Geometry: final body of the model. Coordinates: model frame, mm. A direction names the side the tool comes from. Give positions to 0.01 mm unless a question says otherwise; leave off trailing zeros. Loops run counter-clockwise (first coordinate to the right, second up) from the corner with the lowest first, then second, coordinate; pieces in that order, holes last.
Autodesk Inventor part; units mm, degrees
ref_plane "YZ Plane" through (0, 0, 0) normal (1, 0, 0) x (0, 1, 0)
ref_plane "XZ Plane" through (0, 0, 0) normal (0, 1, 0) x (-1, 0, 0)
ref_plane "XY Plane" through (0, 0, 0) normal (0, 0, 1) x (1, 0, 0)
sketch "スケッチ1" plane through (0, 0, 0) normal (0, 0, 1) x (1, 0, 0)
  line L0 (7.25, -16) -> (-7.25, -16)
  line L1 (-16.25, -16) -> (-16.25, 16)
  line L2 (-7.25, 16) -> (7.25, 16)
  line L3 (16.25, -16) -> (-16.25, 16) construction
  line L4 (-16.25, -16) -> (16.25, 16) construction
  line L5 (16.25, 0) -> (46.25, 0) construction
  line L6 (46.25, -10.5) -> (16.25, -10.5) construction
  line L7 (16.25, 10.5) -> (46.25, 10.5) construction
  line L8 (46.25, 10.5) -> (46.25, -10.5) construction
  line L9 (46.25, -10.5) -> (16.25, 10.5) construction
  line L10 (16.25, -10.5) -> (46.25, 10.5) construction
  line L11 (46.25, 11.5) -> (15.25, 11.5)
  line L12 (15.25, 11.5) -> (15.25, -11.5)
  line L13 (15.25, -11.5) -> (46.25, -11.5)
  line L14 (46.25, 19.5) -> (7.25, 19.5)
  line L15 (7.25, -19.5) -> (46.25, -19.5)
  line L16 (46.25, 11.5) -> (46.25, 19.5)
  line L17 (46.25, -11.5) -> (46.25, -19.5)
  line L18 (16.25, 10.5) -> (16.25, -10.5) construction
  line L19 (7.25, 19.5) -> (7.25, 16)
  line L20 (7.25, -16) -> (7.25, -19.5)
  line L21 (-16.25, -16) -> (-16.25, -26)
  line L22 (-16.25, -26) -> (-7.25, -26)
  line L23 (-7.25, 26) -> (-16.25, 26)
  line L24 (-16.25, 26) -> (-16.25, 16)
  line L25 (-11.75, 26) -> (-11.75, -26) construction
  line L26 (-11.75, 0) -> (-16.25, 0) construction
  circle A0 centre (-11.75, -21) radius 1.6
  line L27 (-7.25, -26) -> (-7.25, -16)
  line L28 (-7.25, 16) -> (-7.25, 26)
  circle A1 centre (-11.75, 21) radius 1.6
  line L29 (46.25, 10.5) -> (16.25, 10.5) construction
  line L30 (31.25, 10.5) -> (31.25, 19.5) construction
  line L31 (31.25, 15) -> (46.25, 15) construction
  circle A2 centre (37.05, 15) radius 1.6 construction
  circle A3 centre (42.25, 15) radius 1.6
  circle A4 centre (25.45, 15) radius 1.6 construction
  circle A5 centre (20.25, 15) radius 1.6
  circle A6 centre (37.05, -15) radius 1.6 construction
  circle A7 centre (42.25, -15) radius 1.6
  circle A8 centre (25.45, -15) radius 1.6 construction
  circle A9 centre (20.25, -15) radius 1.6
  point P0 (0, 0)
  point P1 (31.25, 0)
  dimension "d21" = 32.5
  dimension "d22" = 32
  dimension "d24" = 30
  dimension "d25" = 21
  dimension "d26" = 1
  dimension "d28" = 30
  dimension "d30" = 9
  dimension "d32" = 9
  dimension "d33" = 3.2
  dimension "d34" = 5
  dimension "d35" = 10
  dimension "d36" = 8
  dimension "d37" = 31
  dimension "d38" = 3.5
  dimension "d39" = 35.5
  dimension "d40" = 9
  dimension "d41" = 3.2
  dimension "d42" = 3.2
  dimension "d43" = 4
  dimension "d44" = 31
  dimension "d46" = 2
extrude "押し出し1" add sketch "スケッチ1" along normal blind 3
fillet "フィレット1" radius 2 10 edges at (7.25, 19.5, 1.5) (-7.25, 26, 1.5) (-16.25, 26, 1.5) (46.25, 19.5, 1.5) (46.25, 11.5, 1.5) (46.25, -11.5, 1.5) (46.25, -19.5, 1.5) (7.25, -19.5, 1.5) (-7.25, -26, 1.5) (-16.25, -26, 1.5)
fillet "フィレット2" radius 3 6 edges at (15.25, -11.5, 1.5) (15.25, 11.5, 1.5) (7.25, 16, 1.5) (7.25, -16, 1.5) (-7.25, -16, 1.5) (-7.25, 16, 1.5)
sketch "スケッチ2" plane through (0, 0, 3) normal (0, 0, 1) x (1, 0, 0)
  arc A0 (-16.25, -24) -> (-14.25, -26) centre (-14.25, -24) ccw
  line L0 (-14.25, -26) -> (-9.25, -26)
  arc A1 (-9.25, -26) -> (-7.25, -24) centre (-9.25, -24) ccw
  line L1 (-7.25, -24) -> (-7.25, -19)
  arc A2 (-4.25, -16) -> (-7.25, -19) centre (-4.25, -19) ccw
  line L2 (-4.25, -16) -> (4.4803, -16)
  arc A3 (7.3421, -18.1) -> (4.4803, -16) centre (4.4803, -19) ccw
  arc A4 (7.3421, -18.1) -> (9.25, -19.5) centre (9.25, -17.5) ccw
  line L3 (9.25, -19.5) -> (44.25, -19.5)
  arc A5 (44.25, -19.5) -> (46.25, -17.5) centre (44.25, -17.5) ccw
  line L4 (46.25, -17.5) -> (46.25, -13.5)
  arc A6 (46.25, -13.5) -> (44.25, -11.5) centre (44.25, -13.5) ccw
  line L5 (44.25, -11.5) -> (18.25, -11.5)
  arc A7 (15.25, -8.5) -> (18.25, -11.5) centre (18.25, -8.5) ccw
  line L6 (15.25, -8.5) -> (15.25, 8.5)
  arc A8 (18.25, 11.5) -> (15.25, 8.5) centre (18.25, 8.5) ccw
  line L7 (18.25, 11.5) -> (44.25, 11.5)
  arc A9 (44.25, 11.5) -> (46.25, 13.5) centre (44.25, 13.5) ccw
  line L8 (46.25, 13.5) -> (46.25, 17.5)
  arc A10 (46.25, 17.5) -> (44.25, 19.5) centre (44.25, 17.5) ccw
  line L9 (44.25, 19.5) -> (9.25, 19.5)
  arc A11 (9.25, 19.5) -> (7.3421, 18.1) centre (9.25, 17.5) ccw
  arc A12 (4.4803, 16) -> (7.3421, 18.1) centre (4.4803, 19) ccw
  line L10 (4.4803, 16) -> (-4.25, 16)
  arc A13 (-7.25, 19) -> (-4.25, 16) centre (-4.25, 19) ccw
  line L11 (-7.25, 19) -> (-7.25, 24)
  arc A14 (-7.25, 24) -> (-9.25, 26) centre (-9.25, 24) ccw
  line L12 (-9.25, 26) -> (-14.25, 26)
  arc A15 (-14.25, 26) -> (-16.25, 24) centre (-14.25, 24) ccw
  line L13 (-16.25, 24) -> (-16.25, -24)
  circle A16 centre (42.25, -15) radius 1.6
  circle A17 centre (20.25, -15) radius 1.6
  circle A18 centre (20.25, 15) radius 1.6
  circle A19 centre (42.25, 15) radius 1.6
  circle A20 centre (-11.75, 21) radius 1.6
  circle A21 centre (-11.75, -21) radius 1.6
  circle A22 centre (-11.75, 21) radius 4.6
  circle A23 centre (-11.75, -21) radius 4.6
  line L14 (4.4803, -13) -> (-4.25, -13)
  arc A24 (-9.8384, -16.816) -> (-10.25, -19) centre (-4.25, -19) ccw
  line L15 (-10.25, -19) -> (-10.25, -23)
  line L16 (-10.25, -23) -> (-13.25, -23)
  line L17 (-13.25, 23) -> (-10.25, 23)
  line L18 (-10.25, 23) -> (-10.25, 19)
  arc A25 (-10.25, 19) -> (-9.8384, 16.816) centre (-4.25, 19) ccw
  line L19 (-4.25, 13) -> (4.4803, 13)
  line L20 (9.9347, 16.5) -> (43.25, 16.5)
  line L21 (43.25, 16.5) -> (43.25, 14.5)
  line L22 (43.25, 14.5) -> (18.25, 14.5)
  line L23 (12.25, 8.5) -> (12.25, -8.5)
  arc A26 (14.6318, -13.2863) -> (18.25, -14.5) centre (18.25, -8.5) ccw
  line L24 (18.25, -14.5) -> (43.25, -14.5)
  line L25 (43.25, -14.5) -> (43.25, -16.5)
  line L26 (43.25, -16.5) -> (9.9347, -16.5)
  circle A27 centre (20.25, 15) radius 4.6
  line L27 (-4.25, 13) -> (-11.149, 13)
  line L28 (-4.25, -13) -> (-11.149, -13)
  line L29 (12.25, -8.5) -> (12.25, -10.8578)
  line L30 (12.25, 8.5) -> (12.25, 10.8578)
  line L31 (-13.25, 13) -> (12.25, -13) construction
  line L32 (12.25, 13) -> (-13.25, -13) construction
  line L33 (-13.25, 14.5) -> (-13.25, 23)
  line L34 (4.4803, 13) -> (10.149, 13)
  arc A28 (18.25, 14.5) -> (15.7685, 13.9628) centre (18.25, 8.5) ccw
  line L35 (-13.25, -23) -> (-13.25, -16.6514)
  line L36 (-13.25, -10.8578) -> (-13.25, 10.8578)
  line L37 (10.149, 13) -> (-0.5, 2.1422)
  line L38 (-2.601, 0) -> (-13.25, -10.8578)
  line L39 (-11.149, -13) -> (-0.5, -2.1422)
  line L40 (1.601, 0) -> (12.25, 10.8578)
  line L41 (-13.25, 10.8578) -> (-2.601, 0)
  line L42 (-0.5, -2.1422) -> (10.149, -13)
  line L43 (12.25, -10.8578) -> (1.601, 0)
  line L44 (-0.5, 2.1422) -> (-11.149, 13)
  line L45 (4.4803, -13) -> (10.149, -13)
  arc A29 (9.9347, -16.5) -> (9.3557, -15.5028) centre (4.4803, -19) ccw
  point P0 (0, 0)
  point P1 (-0.5, 0)
  point P2 (-0.5, 0)
  dimension "d51" = 3
  dimension "d52" = 3
  dimension "d53" = 3
  dimension "d54" = 3
extrude "押し出し2" cut sketch "スケッチ2" against normal through all contours L14 L28 L39 L42 L45 | L19 L34 L37 L44 L27 | L23 L29 L43 L40 L30 | L36 L41 L38
fillet "フィレット3" radius 3 12 edges at (-11.149, 13, 1.5) (10.149, 13, 1.5) (-0.5, 2.1422, 1.5) (-13.25, 10.8578, 1.5) (-13.25, -10.8578, 1.5) (-2.601, 0, 1.5) (-0.5, -2.1422, 1.5) (-11.149, -13, 1.5) (10.149, -13, 1.5) (1.601, 0, 1.5) (12.25, 10.8578, 1.5) (12.25, -10.8578, 1.5)
properties part number "肩ピッチ固定板_アルミ(A2017)_t3" material "アルミニウム 2014-T6"
Item 1: Section query B-B on x = 20.25. Return loops of the section in (y, z), plus the area to 3 significant figures.
Values follow:
outline: (-19.5, 0) - (-16.6, 0) - (-16.6, 3) - (-19.5, 3) - close; (-13.4, 0) - (-11.5, 0) - (-11.5, 3) - (-13.4, 3) - close; (11.5, 0) - (13.4, 0) - (13.4, 3) - (11.5, 3) - close; (16.6, 0) - (19.5, 0) - (19.5, 3) - (16.6, 3) - close
area: 28.8 mm2
Item 2: Section query D-D on z = 1.85. Give the number of separate pieces and of enclosed holes in the cut face, plus the area to 3 significant figures.
Values follow:
separate pieces: 1
enclosed holes: 10
area: 1,330 mm2
Item 3: Section query C-C on y = 10. Return loops of the section in (x, z).
Values follow:
outline: (-16.25, 0) - (-7, 0) - (-7, 3) - (-16.25, 3) - close; (6, 0) - (15.65, 0) - (15.65, 3) - (6, 3) - close
Item 4: Ray query, probe 1 along Y at (x, z) = (42.25, 1.95); probe 2 along Y at (x, z) = (32, 2.8); probe 3 along Y at (x, z) = (-11.75, 2). Return the intervals inside material, ascending.
Values follow:
probe 1: y = -19.5 to -16.6, -13.4 to -11.5, 11.5 to 13.4, 16.6 to 19.5
probe 2: y = -19.5 to -11.5, 11.5 to 19.5
probe 3: y = -26 to -22.6, -19.4 to -6.11, 6.11 to 19.4, 22.6 to 26
Item 5: Section query A-A on x = 38.5. Return loops of the section in (y, z).
Values follow:
outline: (-19.5, 0) - (-11.5, 0) - (-11.5, 3) - (-19.5, 3) - close; (11.5, 0) - (19.5, 0) - (19.5, 3) - (11.5, 3) - close
Item 6: Pin query (flat end, axial travel): pin 1 (1.5 mm diameter, centred on x = 2, z = 2, fed in from +Y); pin 2 (4 mm diameter, centred on x = 42.25, y = -15, fed in from -Z); pin 3 (0.9 mm diameter, centred on y = 0, z = 2, fed in from +X); pin 4 (0.9 mm diameter, centred on x = 34.5, z = 1, fed in from -Y). Return the tip coordinate at first contact, or that it passes through.
Values follow:
pin 1: stops at y = 16
pin 2: stops at z = 0
pin 3: stops at x = 15.25
pin 4: stops at y = -19.5
Item 7: Set-up query: faces 1 (the face through (3.37, -6.09, 1.52)), 2 (the face through (45.65, 12.07, 1.52)), 3 (the face through (27, -19.5, 1)). Return all of +Z, -Z, +X, -X, +Y, -Y with unobstructed straight access to the full face (end or side cutting, diameter ignored); none if empty.
Values follow:
face 1: +Z, -Z
face 2: +Z, -Z, +X
face 3: +Z, -Z, +X, -Y
Item 8: Draft query along X for faces 4 (the face through (0, -13, 2)), 5 (the face through (46.25, -15, 1)), 6 (the face through (31, -11.5, 1)), 7 (the face through (-3.803, 0.033, 1.479)). Return one class per face: +X half, -X half, draft (parallel to the pull), parting line (faces both ways), or undercut.
Values follow:
face 4: undercut
face 5: +X half
face 6: draft
face 7: undercut
